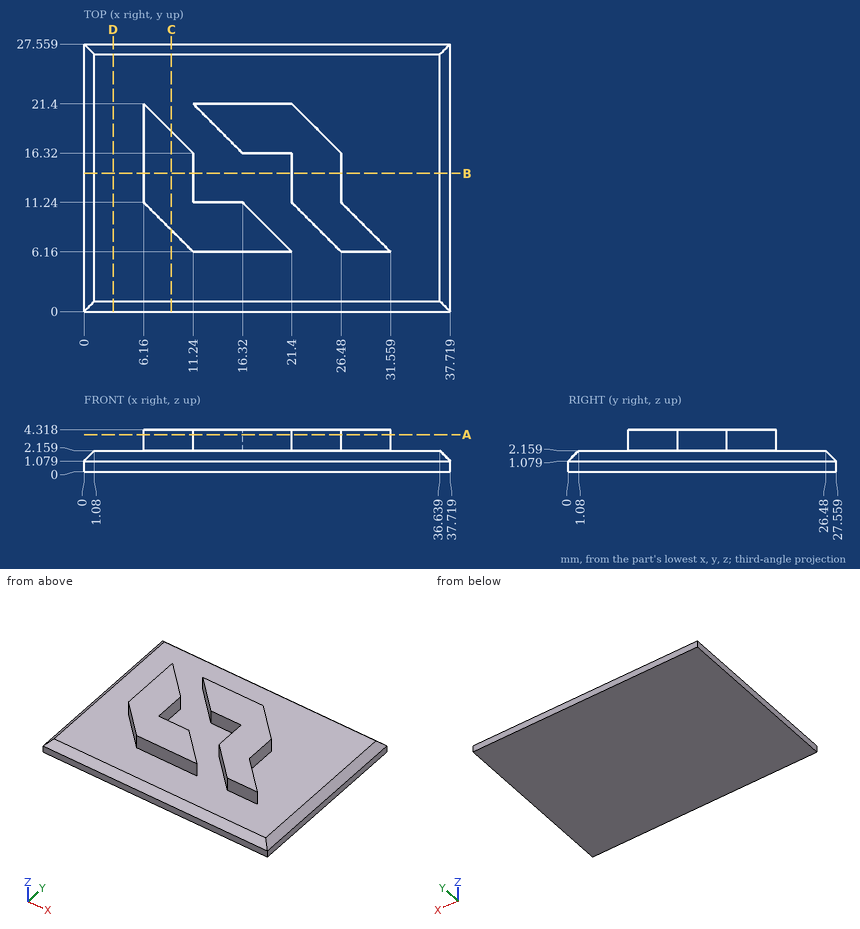
Input: dimensioned drawing with shaded views. Units: mm. Origin: part minimum x, y, z. Coordinates: 2 decimals unless noted, no trailing zeros. Loops run counter-clockwise (first coordinate to the right, second up) from the corner with the lowest first, then second, coordinate; pieces in that order, holes last. Notation, with made-up numbers: M 8,-31 L 61,-31 A21 cw 61,-9 Z; hole C -30.75,60.25 d11. An arc over 180 degrees is marked long. Use a Markdown table: item, result. Add a question column.
Q1. Section query B-B, the plane y = 14.25. Return loops of the section in (x, z), and give its area (3 significant figures).
Q2. First-contact query: pin 1 (1.1 mm diameter, centred on x = 16, z = 3, fed in from +Y); pin 2 (1.7 mm diameter, centred on x = 29.5, z = 3.5, fed in from -Y); pin 3 (2.5 mm diameter, centred on x = 19, z = 2.5, fed in from -Y). Flat tips, straight axial feed; report the tip coordinate or a pass-through.
Q3. Section query C-C, the plane x = 9. Return loops of the section in (y, z).
Q4. Section query A-A, the plane z = 3.8. Return loops of the section in (x, y).
Q5. Section query D-D, the plane x = 3. Return loops of the section in (y, z).
Q6. Material intervals for L1, parallel to Z at x = 35, y = 19; L2, parallel to Y at x = 16, z = 2.3; L3, parallel to X at y = 8.75, z = 2.9, sorted ascending.
Result:
| question | item | result |
|---|---|---|
| 1 | outline | M 0,0 L 37.72,0 L 37.72,1.08 L 36.64,2.16 L 26.48,2.16 L 26.48,4.32 L 21.4,4.32 L 21.4,2.16 L 11.24,2.16 L 11.24,4.32 L 6.16,4.32 L 6.16,2.16 L 1.08,2.16 L 0,1.08 Z |
| 1 | area | 102 mm2 |
| 2 | pin 1 | stops at y = 21.4 |
| 2 | pin 2 | stops at y = 6.16 |
| 2 | pin 3 | stops at y = 0.17 |
| 3 | outline | M 0,0 L 27.56,0 L 27.56,1.08 L 26.48,2.16 L 18.56,2.16 L 18.56,4.32 L 8.4,4.32 L 8.4,2.16 L 1.08,2.16 L 0,1.08 Z |
| 4 | outline | M 6.16,11.24 L 11.24,6.16 L 21.4,6.16 L 16.32,11.24 L 11.24,11.24 L 11.24,16.32 L 6.16,21.4 Z; M 11.24,21.4 L 16.32,16.32 L 21.4,16.32 L 21.4,11.24 L 26.48,6.16 L 31.56,6.16 L 26.48,11.24 L 26.48,16.32 L 21.4,21.4 Z |
| 5 | outline | M 0,0 L 27.56,0 L 27.56,1.08 L 26.48,2.16 L 1.08,2.16 L 0,1.08 Z |
| 6 | L1 | z = 0 to 2.16 |
| 6 | L2 | y = 6.16 to 11.24, 16.64 to 21.4 |
| 6 | L3 | x = 8.65 to 18.81, 23.89 to 28.97 |
